For this review, use the dimensioned drawing (mm, ordinates from the lowest corner) and the shaded views. A direction names the side the tool comes from. Coordinates: 2 decimals unless noted, no trailing zeros. Loops run counter-clockwise (first coordinate to the right, second up) from the corner with the lowest first, then second, coordinate; pieces in that order, holes last. Notation, with made-up numbers: (81.25, 44.5) - (96.25, 44.5) arc R23 cw to (96.25, 74.5) - close; hole circle Ø6 at (46.5, 20.25). An arc over 180 degrees is marked (long way). Use one line per item in the form item = value. Start each with the question number.
(1) Add section D-D (z = 1.25). State the section outline as (x, y) points, plus the area to 3 significant figures.
(2) Clearance check with flat-ended pins moving along their axes: pin 1 Ø2.5 at (x, y) = (2, 2) entering from +Z; pin 2 Ø1.8 at (x, y) = (2.5, 2.5) entering from -Z; pin 3 Ø1.5 at (x, z) = (1, 6) entering from +Y (3 decimals). State where each tip first meets the part, or that it passes through.
(3) Add section C-C (y = 4.05). State the section outline as (x, z) points, plus the area to 3 significant figures.
(4) Add section B-B (x = 1.2). State the section outline as (y, z) points.
(5) Add section A-A (z = 3.5). State the section outline as (x, y) points, plus the area to 3 significant figures.
(6) Tool access review of the marked faces 4, 5 and 6: name each direction out of +Z, -Z, +X, -X, +Y, -Y from which nothing blocks a thin tool from reaching the whole face with its end or side.
(7) For L1, parallel to Y at x = 2.5, z = 0.4; L2, parallel to Z at x = 2.25, y = 3.9; L3, parallel to Y at x = 2.6, z = 1.25 (1 decimal), list the stretches that pass through material, from the lowest coordinate up.
(8) The part is to be moulded in two halves that separate along X. For the marked faces 1, 2 and 3, say which applies: pulls with the +X half, pulls with the -X half, needs draft (parallel to the pull), parting line crosses it, or undercut.
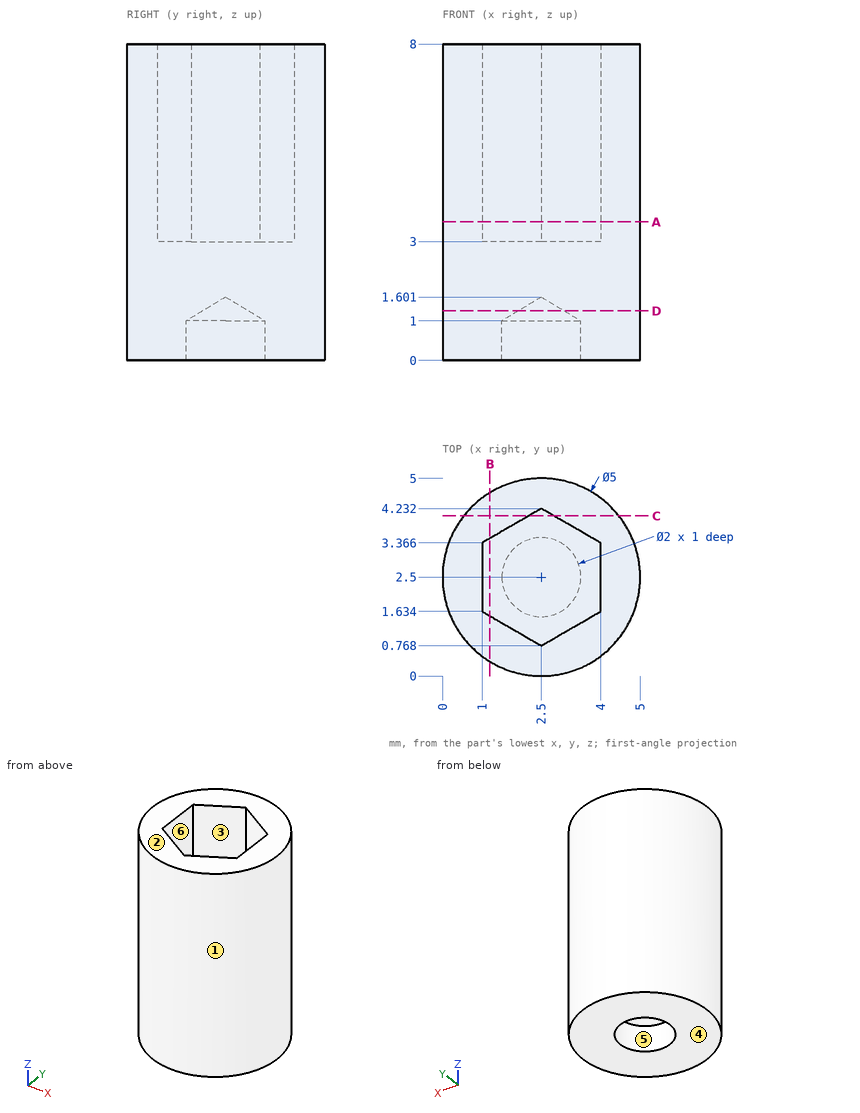
Computed values:
q1.outline = circle Ø5 at (2.5, 2.5); hole circle Ø1.17 at (2.5, 2.5)
q1.area = 18.6 mm^2
q2.pin_1 = 8
q2.pin_2 = 1.06
q2.pin_3 = 4.885
q3.outline = (0.54, 0) - (4.46, 0) - (4.46, 8) - (2.82, 8) - (2.82, 3) - (2.18, 3) - (2.18, 8) - (0.54, 8) - close
q3.area = 28.2 mm^2
q4.outline = (0.36, 0) - (4.64, 0) - (4.64, 8) - (3.48, 8) - (3.48, 3) - (1.52, 3) - (1.52, 8) - (0.36, 8) - close
q5.outline = circle Ø5 at (2.5, 2.5); hole (1, 1.63) - (2.5, 0.77) - (4, 1.63) - (4, 3.37) - (2.5, 4.23) - (1, 3.37) - close
q5.area = 11.8 mm^2
q6.face_4 = -Z, +X, -X, +Y, -Y
q6.face_5 = -Z
q6.face_6 = +Z
q7.L1 = 0 to 1.5, 3.5 to 5
q7.L2 = 0 to 3
q7.L3 = 0 to 1.9, 3.1 to 5
q8.face_1 = parting line crosses it
q8.face_2 = needs draft
q8.face_3 = undercut
